Autodesk Fusion 360 part; units mm, degrees
sketch "Sketch1" plane through (0, 0, 0) normal (0, 0, 1) x (1, 0, 0)
  circle A0 centre (0, 0) radius 3.1
  line L0 (-0.4, 3.1) -> (0.4, 3.1)
  line L1 (0.4, 3.1) -> (0.4, -3.1)
  line L2 (0.4, -3.1) -> (-0.4, -3.1)
  line L3 (-0.4, -3.1) -> (-0.4, 3.1)
  line L4 (0, 0) -> (0, 3.1)
  circle A1 centre (0, 0) radius 5
  dimension "d1" = 6.2
  dimension "d2" = 0.8
  dimension "d3" = 6.2
  dimension "d4" = 10
extrude "Extrude1" add sketch "Sketch1" along normal blind 7 contours A0 L1 L3 | A0 L0 L1 | A0 L1 L2 | A0 L0 L3 | A0 L2 L3 | A1
sketch "Sketch2" plane through (0, 0, 0) normal (0, 0, 1) x (1, 0, 0)
  circle A0 centre (0, 0) radius 12.5
  circle A1 centre (0, -12.5) radius 1.5
  circle A2 centre (5.4235, -11.2621) radius 1.5
  circle A3 centre (9.7729, -7.7936) radius 1.5
  circle A4 centre (12.1866, -2.7815) radius 1.5
  circle A5 centre (12.1866, 2.7815) radius 1.5
  circle A6 centre (9.7729, 7.7936) radius 1.5
  circle A7 centre (5.4235, 11.2621) radius 1.5
  circle A8 centre (0, 12.5) radius 1.5
  circle A9 centre (-5.4235, 11.2621) radius 1.5
  circle A10 centre (-9.7729, 7.7936) radius 1.5
  circle A11 centre (-12.1866, 2.7815) radius 1.5
  circle A12 centre (-12.1866, -2.7815) radius 1.5
  circle A13 centre (-9.7729, -7.7936) radius 1.5
  circle A14 centre (-5.4235, -11.2621) radius 1.5
  circle A15 centre (0, 0) radius 5
  line L0 (12.5, 0.6) -> (5.5, 0.6)
  line L1 (5.5, 0.6) -> (5.5, -0.6)
  line L2 (5.5, -0.6) -> (12.5, -0.6)
  line L3 (12.5, -0.6) -> (12.5, 0.6)
  line L4 (0, 0) -> (12.5, 0)
  dimension "d7" = 25
  dimension "d8" = 3
  dimension "d10" = 360
  dimension "d13" = 10
  dimension "d16" = 7
  dimension "d17" = 1.2
extrude "Extrude2" add sketch "Sketch2" against normal blind 5 contours A0 L0 L1 L4 | A0 L1 L2 L4 | A15 | A0 A1 A2 A3 A4 A5 A6 A7 A8 A9 A10 A11 A12 A13 A14 L0 L1 L2
extrude "Extrude3" add sketch "Sketch2" along normal blind 5 contours A0 L0 L1 L4 | A0 L1 L2 L4 | A0 A1 A2 A3 A4 A5 A6 A7 A8 A9 A10 A11 A12 A13 A14 L0 L1 L2
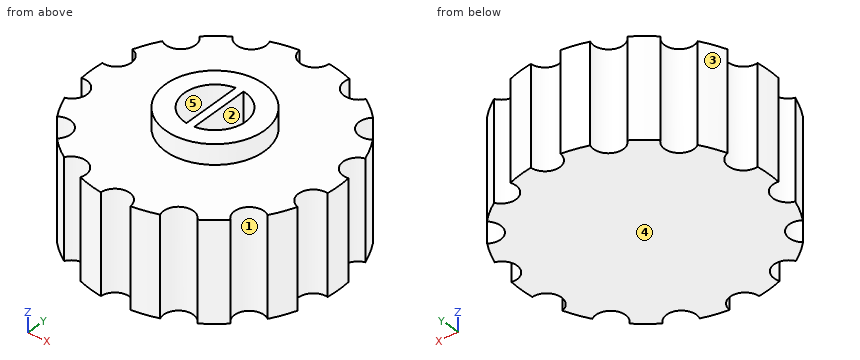
Work out the finished part from the listing and answer in its coordinate system (mm). Face numbers are marked on the shaded views. A direction names the side the tool comes from. Coordinates: 2 decimals unless noted, no trailing zeros. Loops run counter-clockwise (first coordinate to the right, second up) from the corner with the lowest first, then second, coordinate; pieces in that order, holes last. Notation, with made-up numbers: (37, 84) - (53, 84) arc R32 ccw to (53, 118) - close; hole circle Ø11 at (-11.5, -30). An arc over 180 degrees is marked (long way). Use a Markdown table: item, result.
Item 1: Find section A-A, the plane z = 4. State how many separate pieces and enclosed holes the cut face has, and give its area (3 significant figures).
Evaluation:
| item | result |
|---|---|
| separate pieces | 1 |
| enclosed holes | 2 |
| area | 417 mm2 |
Item 2: The mould has two halves that part along X. Classify the marked faces 3, 4 and 5: +X half, -X half, draft (parallel to the pull), parting line (faces both ways), or undercut.
Evaluation:
| item | result |
|---|---|
| face 3 | -X half |
| face 4 | draft |
| face 5 | undercut |
Item 3: Find section B-B, the plane y = 0. Determine the outline of the cut face in (x, z).
Evaluation:
| item | result |
|---|---|
| outline | (-12.5, -5) - (12.5, -5) - (12.5, 5) - (5, 5) - (5, 7) - (3.1, 7) - (3.1, 0) - (0.4, 0) - (0.4, 7) - (-0.4, 7) - (-0.4, 0) - (-3.1, 0) - (-3.1, 7) - (-5, 7) - (-5, 5) - (-12.5, 5) - close |
Item 4: Given pin 1 Ø2 at (y, z) = (5.5, 0) entering from +X; pin 2 Ø2 at (y, z) = (4.5, -1.5) entering from -X; pin 3 Ø2 at (y, z) = (-9.5, 4) entering from +X, each flat-ended and moving along its own axis, determine where each tip first touches the part or whether it passes through.
Evaluation:
| item | result |
|---|---|
| pin 1 | stops at x = 11.66 |
| pin 2 | stops at x = -11.77 |
| pin 3 | stops at x = 8.77 |
Item 5: Find section D-D, the plane z = -2.5. Determine the outline of the cut face in (x, y), and give its area (3 significant figures).
Evaluation:
| item | result |
|---|---|
| outline | (-12.43, -1.3) arc R1.5 cw to (-11.77, -4.22) arc R12.5 ccw to (-10.64, -6.57) arc R1.5 cw to (-8.77, -8.91) arc R12.5 ccw to (-6.73, -10.53) arc R1.5 cw to (-4.04, -11.83) arc R12.5 ccw to (-1.5, -12.41) arc R1.5 cw to (1.5, -12.41) arc R12.5 ccw to (4.04, -11.83) arc R1.5 cw to (6.73, -10.53) arc R12.5 ccw to (8.77, -8.91) arc R1.5 cw to (10.64, -6.57) arc R12.5 ccw to (11.77, -4.22) arc R1.5 cw to (12.43, -1.3) arc R12.5 ccw to (12.43, 1.3) arc R1.5 cw to (11.77, 4.22) arc R12.5 ccw to (10.64, 6.57) arc R1.5 cw to (8.77, 8.91) arc R12.5 ccw to (6.73, 10.53) arc R1.5 cw to (4.04, 11.83) arc R12.5 ccw to (1.5, 12.41) arc R1.5 cw to (-1.5, 12.41) arc R12.5 ccw to (-4.04, 11.83) arc R1.5 cw to (-6.73, 10.53) arc R12.5 ccw to (-8.77, 8.91) arc R1.5 cw to (-10.64, 6.57) arc R12.5 ccw to (-11.77, 4.22) arc R1.5 cw to (-12.43, 1.3) arc R12.5 ccw to start |
| area | 443 mm2 |
Item 6: For the marked faces 1 and 2, determine the directions among +Z, -Z, +X, -X, +Y, -Y from which every point of the face is accessible in a straight line to the end or side of a thin tool.
Evaluation:
| item | result |
|---|---|
| face 1 | +Z, -Z |
| face 2 | +Z |
Item 7: Consider probe 1 along X at (y, z) = (10, -0.75); probe 2 along X at (y, z) = (2.25, 3); probe 3 along Z at (x, y) = (8.25, -1.5). Determine where each line is inside the solid, lowest interval first. Write a range as from..to.
Evaluation:
| item | result |
|---|---|
| probe 1 | x = -7.5..-6.23, -4.61..4.61, 6.23..7.5 |
| probe 2 | x = -10.78..-2.13, -0.4..0.4, 2.13..10.78 |
| probe 3 | z = -5..5 |
Item 8: Find section C-C, the plane x = 0. Determine the outline of the cut face in (y, z).
Evaluation:
| item | result |
|---|---|
| outline | (-11, -5) - (11, -5) - (11, 5) - (5, 5) - (5, 7) - (-5, 7) - (-5, 5) - (-11, 5) - close |
